Autodesk Inventor part; units mm, degrees
ref_plane "YZ Plane" through (0, 0, 0) normal (1, 0, 0) x (0, 1, 0)
ref_plane "XZ Plane" through (0, 0, 0) normal (0, 1, 0) x (-1, 0, 0)
ref_plane "XY Plane" through (0, 0, 0) normal (0, 0, 1) x (1, 0, 0)
sketch "Sketch3" plane through (0, 0, 0) normal (0, 1, 0) x (-1, 0, 0)
  line L0 (0, 0) -> (5, 0)
  line L1 (31.8661, -24.4237) -> (31.8661, -64.4237)
  line L2 (41.8661, -64.4237) -> (41.8661, -20)
  line L3 (0, 10) -> (0, 0)
  line L4 (8.8661, 10) -> (41.8661, -20)
  line L5 (31.8661, -24.4237) -> (5, 0)
  line L6 (8.8661, 10) -> (0, 10)
  line L7 (5, 0) -> (0, 0)
  line L8 (31.8661, -24.4237) -> (31.8661, -64.4237)
  line L9 (41.8661, -64.4237) -> (41.8661, -20)
  line L10 (5, 0) -> (0, 0)
  arc A0 (31.8661, -64.4237) -> (41.8661, -64.4237) centre (36.8661, -64.4237) ccw
  circle A1 centre (0, -35.9984) radius 30
  point P0 (31.8661, -44.4237)
  point P1 (0, 5)
  dimension "d51" = 10
  dimension "d56" = 10
  dimension "d57" = 30
  dimension "d58" = 33
  dimension "d59" = 5
  dimension "d60" = 5
  dimension "d61" = 40
  dimension "d64" = 10
  dimension "d65" = 10
  dimension "d66" = 60
extrude "Extrusion2" add sketch "Sketch3" along normal blind 3 contours L3 L6 L4 L2 A0 L1 L5 L0
sketch "Sketch4" plane through (0, 3, 0) normal (0, 1, 0) x (1, 0, 0)
  line L0 (0, -10) -> (0, 0)
  arc A0 (-31.8661, 64.4237) -> (-41.8661, 64.4237) centre (-36.8661, 64.4237) ccw
  point P0 (-6.55, -5)
  point P1 (0, -5)
  point P2 (-36.8661, 69.4237)
  dimension "d77" = 6.55
hole "Hole2" at (-6.55, 3, 5) at (-36.8661, 3, -64.4237) direction (0, -1, 0) diameter 3.2 end through all
fillet "Fillet1" radius 5 4 edges at (-8.8661, 1.5, 10) (-41.8661, 1.5, -20) (-31.8661, 1.5, -24.4237) (-5, 1.5, 0)
mirror "Mirror3" about plane through (0, 0, 10) normal (1, 0, 0) of "Extrusion2", "Hole2", "Fillet1"
properties part number "Claw4" material "Copper, Cast"
The listing builds one solid part. Answer for the finished solid, in the listing's coordinates (mm). A direction names the side the tool comes from. Give positions to 0.01 mm unless a question says otherwise; leave off trailing zeros. Order: outer loops, then holes, each group sorted by start corner. A loop starts at its lowest first (then second) coordinate and runs counter-clockwise, first axis right, second up. Notation, with made-up numbers: (-38, 79.25) -> (13, 79.25) arc R24 cw to (13, 112.25) -> close; hole circle Ø6 at (40.5, 32). An arc over 180 degrees is marked (long way). Answer as a JSON object with one key per item and string values. Group by question number.
Item 1: The part is cut by section A-A on z = -35. Write down the section's boundary in (x, y).
Item 2: Consider L1, parallel to X at y = 1.1, z = -41.5; L2, parallel to X at y = 1.4, z = 5; L3, parallel to X at y = 0.45, z = -13.5. Determine where each line is inside the solid, lowest interval first. Write a range as from..to.
Item 3: The part is cut by section C-C on z = 5. Write down the section's boundary in (x, y).
Item 4: The part is cut by section B-B on y = 1.2. Write down the section's boundary in (x, z).
Item 5: The part is cut by section D-D on x = -26. Write down the section's boundary in (y, z), and give its area (3 significant figures).
Item 6: Determine the mould class of faces 1 (the flat face through (18.2, 1.5, -12)), 2 (the flat face through (19, 0, -12)), 3 (the cylindrical face through (4.964, 1.479, 4.792)) for opening direction Z: pulls with the +Z half, pulls with the -Z half, needs draft (parallel to the pull), parting line crosses it, or undercut.
Item 7: A tool of negligible diameter and unlimited length cuts with its end or side. For faces 4 (the flat face through (0, 1, 0)), 5 (the flat face through (41.866, 1, -43)), from which of +Z, -Z, +X, -X, +Y, -Y can it reach the whole face along a straight path? Write none if from no direction.
Result set:
{
 "1": {"outline": "(-41.87, 0) -> (-31.87, 0) -> (-31.87, 3) -> (-41.87, 3) -> close; (31.87, 0) -> (41.87, 0) -> (41.87, 3) -> (31.87, 3) -> close"},
 "2": {"L1": "-41.87..-31.87, 31.87..41.87", "L2": "-14.37..-8.15, -4.95..4.95, 8.15..14.37", "L3": "-34.72..-19.85, 19.85..34.72"},
 "3": {"outline": "(-14.37, 0) -> (-8.15, 0) -> (-8.15, 3) -> (-14.37, 3) -> close; (-4.95, 0) -> (4.95, 0) -> (4.95, 3) -> (-4.95, 3) -> close; (8.15, 0) -> (14.37, 0) -> (14.37, 3) -> (8.15, 3) -> close"},
 "4": {"outline": "(-41.87, -64.42) arc R5 ccw to (-31.87, -64.42) -> (-31.87, -26.64) arc R5 cw to (-30.23, -22.94) -> (-6.43, -1.3) arc R5 cw to (-3.07, 0) -> (3.07, 0) arc R5 cw to (6.43, -1.3) -> (30.23, -22.94) arc R5 cw to (31.87, -26.64) -> (31.87, -64.42) arc R5 ccw to (41.87, -64.42) -> (41.87, -22.21) arc R5 ccw to (40.23, -18.51) -> (10.3, 8.7) arc R5 ccw to (6.93, 10) -> (-6.93, 10) arc R5 ccw to (-10.3, 8.7) -> (-40.23, -18.51) arc R5 ccw to (-41.87, -22.21) -> close; hole circle Ø3.2 at (-36.87, -64.42); hole circle Ø3.2 at (-6.55, 5); hole circle Ø3.2 at (6.55, 5); hole circle Ø3.2 at (36.87, -64.42)"},
 "5": {"outline": "(0, -19.09) -> (3, -19.09) -> (3, -5.58) -> (0, -5.58) -> close", "area": "40.5 mm²"},
 "6": {"face 1": "pulls with the -Z half", "face 2": "needs draft", "face 3": "undercut"},
 "7": {"face 4": "-Z, +Y, -Y", "face 5": "+Z, -Z, +X, +Y, -Y"}
}
